```python
from build123d import *

# Parameters (mm, degrees)
F0_W     = 200
F0_H     = 150
F1_DEPTH = 25
F2_R     = 50
F5_SIZE  = 10
F6_R     = 9.7838698058
F6_R_2   = 10
F6_R_3   = 10.147546669
F6_R_4   = 9.9344737349
F7_DEPTH = 25


with BuildPart() as f1:
    # F0 (on Top) → F1 (new body, symmetric)
    with BuildSketch(Plane.XY):
        Rectangle(F0_W, F0_H)
    extrude(amount=F1_DEPTH, both=True)

    # F2
    f2_edges = [f1.edges().sort_by_distance(p)[0] for p in [
        (-100, -75, 0),
        (100, -75, 0),
        (100, 75, 0),
        (-100, 75, 0),
    ]]
    fillet(f2_edges, radius=F2_R)

    # F3 (on Front) → F4 (revolve, cut)
    with BuildSketch(Plane.XZ):
        with BuildLine():
            Line((0, 25), (-58.1593476236, 25))
            add(Edge.make_bspline(
                [(-58.1593476236, 25), (-53.9096311875, 12.7192745819), (-17.6634682668, 23.9500074163), (-23.8563775859, 5.5907417856), (0, 6.6510247998)],
                knots=[0, 0, 0, 0, 0.5060175337, 1, 1, 1, 1], degree=3))
            Line((0, 6.6510247998), (0, 25))
        make_face()
    revolve(axis=Axis((0, 0, 15.8255123999), (0, 0, 1)), mode=Mode.SUBTRACT)

    # F5
    f5_edges = [f1.edges().sort_by_distance(p)[0] for p in [
        (0, -75, 25),
    ]]
    chamfer(f5_edges, length=F5_SIZE)

    # F6 (on face) → F7 (cut)
    with BuildSketch(Plane.XY.offset(25)):
        with Locations((-25.5249421373, 0)):
            Circle(F6_R)
        with Locations((0, 25.7132698898)):
            Circle(F6_R_2)
        with Locations((25.905932002, 0)):
            Circle(F6_R_3)
        with Locations((0, -24.9556606683)):
            Circle(F6_R_4)
    extrude(amount=-F7_DEPTH, mode=Mode.SUBTRACT)


solid = f1.part
```
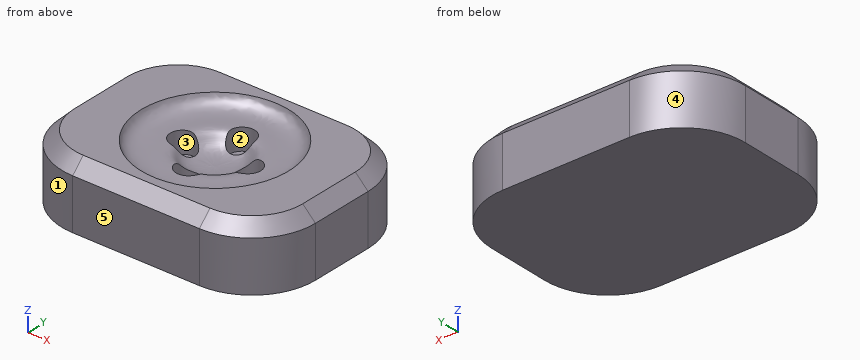
Part model, mm, in its own coordinate system. Face numbers are marked on the shaded views. A direction names the side the tool comes from. Round coordinates to 2 decimals unless told otherwise and drop trailing zeros. Loops run counter-clockwise (first coordinate to the right, second up) from the corner with the lowest first, then second, coordinate; pieces in that order, holes last.
Item 1: Drill centre lines: line 1 (Y direction, x = 0, z = 4); line 2 (Y direction, x = 0, z = 12.75); line 3 (Y direction, x = -25.5, z = 12.5). Where is each one in solid material? Low to high.
Item 2: 3-axis set-ups, long thin cutter, end or side, ignore diameter. For the marked faces 1 and 2: which of +Z, -Z, +X, -X, +Y, -Y reach the whole face in a straight line?
Item 3: Drop flat-ended pins along their axis: P1, Ø4, axis at y = -33, z = 18.5, coming from the -X side; P2, Ø10, axis at x = -30.5, y = 4, coming from the +Z side; P3, Ø1.5, axis at x = 53, z = 18, coming from the -Y side. Give the stop position or say it passes through.
Item 4: Mould opens along X. For the marked faces 3, 4 and 5 say: +X half, -X half, draft (parallel to the pull), parting line (faces both ways), or undercut.
Item 5: Cut at A-A, the plane z = -10.5. Give the cut face in (x, y), then the cut area to 3 significant figures.
A:
1. line 1: y = -75 to -34.89, -15.02 to 15.71, 35.71 to 75
1. line 2: y = -75 to -34.89, 35.71 to 75
1. line 3: y = -75 to -9.78, 9.78 to 75
2. face 1: +Z, -Z, -X, -Y
2. face 2: +Z
3. P1: stops at x = -97.86
3. P2: stops at z = 16.94
3. P3: stops at y = -72.66
4. face 3: undercut
4. face 4: -X half
4. face 5: draft
5. outline: (-100, -25) arc R50 ccw to (-50, -75) - (50, -75) arc R50 ccw to (100, -25) - (100, 25) arc R50 ccw to (50, 75) - (-50, 75) arc R50 ccw to (-100, 25) - close
5. area: 27,900 mm2
